For this review, take the finished solid that the model builds, in its own axes (mm). Give positions to 0.01 mm unless a question says otherwise; leave off trailing zeros. Loops run counter-clockwise (first coordinate to the right, second up) from the corner with the lowest first, then second, coordinate; pieces in that order, holes last. Notation, with made-up numbers: M -8.5,-16.5 L 19.5,-16.5 A26 ccw 19.5,5.5 Z; hole C 80,-38 d1. An arc over 180 degrees is marked long. Use CSV: the item, a comma, the result in double quotes. Start each with the question number.
1. Take a section at B-B, the plane x = 120.5. Write out the cut boundary in (y, z), and give its area (3 significant figures).
2. Insertion check: P1, Ø1, axis at x = 26.5, y = 0, coming from the -Z side. The pin has a flat end and moves straight along its axis. Give the tip position at first contact, or say it passes through.
3. To check wall thickness, follow line 1 (Y direction, x = 22, z = -1.95); line 2 (X direction, y = 1, z = -1.4); line 3 (X direction, y = -1.5, z = -0.3). State the ranges of each line that lie inside material, in increasing order. Write a range as [from, to].
4. Take a section at C-C, the plane y = 0. Write out the cut boundary in (x, z), and give its area (3 significant figures).
5. Take a section at A-A, the plane z = -2.3. Write out the cut boundary in (x, y), and give its area (3 significant figures).
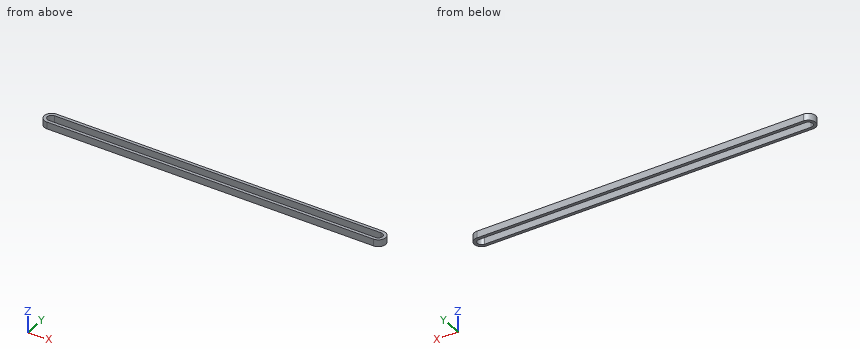
from build123d import *

# Parameters (mm, degrees)
BOSS_EXTRUDE1_DEPTH = 3


with BuildPart() as part:
    # Sketch2 → Boss-Extrude1 (new body)
    with BuildSketch(Plane.XY):
        with BuildLine():
            Line((0, 3.2), (143.6, 3.2))
            ThreePointArc((143.6, 3.2), (146.8, 0), (143.6, -3.2))
            Line((143.6, -3.2), (0, -3.2))
            ThreePointArc((0, -3.2), (-3.2, 0), (0, 3.2))
        make_face()
        with BuildLine():
            Line((0, 1.872), (143.6, 1.872))
            ThreePointArc((143.6, 1.872), (145.472, 0), (143.6, -1.872))
            Line((143.6, -1.872), (0, -1.872))
            ThreePointArc((0, -1.872), (-1.872, 0), (0, 1.872))
        make_face(mode=Mode.SUBTRACT)
    extrude(amount=-BOSS_EXTRUDE1_DEPTH)


solid = part.part
Result set:
1,outline,"M -3.2,-3 L -1.87,-3 L -1.87,0 L -3.2,0 Z; M 1.87,-3 L 3.2,-3 L 3.2,0 L 1.87,0 Z"
1,area,"7.97 mm2"
2,P1,"through"
3,line 1,"[-3.2, -1.87], [1.87, 3.2]"
3,line 2,"[-3.04, -1.58], [145.18, 146.64]"
3,line 3,"[-2.83, -1.12], [144.72, 146.43]"
4,outline,"M -3.2,-3 L -1.87,-3 L -1.87,0 L -3.2,0 Z; M 145.47,-3 L 146.8,-3 L 146.8,0 L 145.47,0 Z"
4,area,"7.97 mm2"
5,outline,"M 0,-3.2 L 143.6,-3.2 A3.2 ccw 143.6,3.2 L 0,3.2 A3.2 ccw Z; hole M 0,-1.87 L 143.6,-1.87 A1.87 ccw 143.6,1.87 L 0,1.87 A1.87 ccw Z"
5,area,"403 mm2"
